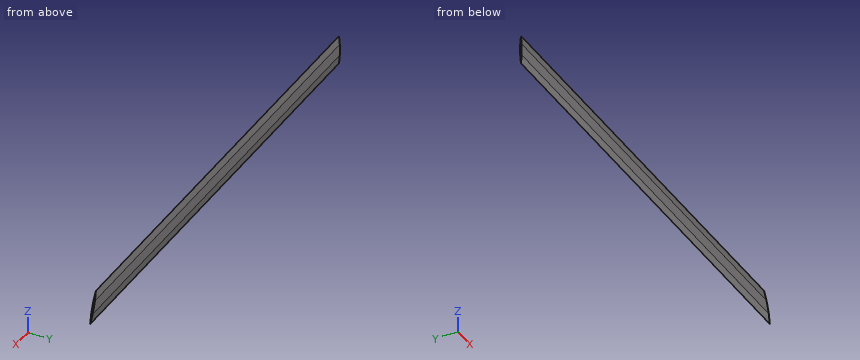
```python
from build123d import *

# Parameters (mm, degrees)
BOSS_EXTRUDE1_DEPTH = 1
CHAMFER1_SIZE       = 0.5
CHAMFER1_SIZE_2     = 6
CHAMFER2_SIZE       = 6
CHAMFER2_SIZE_2     = 0.5


with BuildPart() as part:
    # Sketch1 → Boss-Extrude1 (new body)
    with BuildSketch(Plane(origin=(0, 0, 0), x_dir=(1, 0, 0), z_dir=(0, 1, 0))):
        Polygon((0, -20), (0, 0), (320, 0), (312.720595315, -20), align=None)
    extrude(amount=BOSS_EXTRUDE1_DEPTH)

    # Chamfer1
    # the kernel refuses this chamfer: 6, 0.5 mm, written as the material it takes off along each edge
    with BuildSketch(Plane(origin=(-15.598007041, 0, 0), x_dir=(0, 0.908488621033374, -0.4179095900465534), z_dir=(1, 0, 0))) as chamfer1_piece_1:
        Polygon((CHAMFER1_SIZE * 0.908488621033, CHAMFER1_SIZE * 0.417909590047), (-CHAMFER1_SIZE_2 * 0.417909590047, CHAMFER1_SIZE_2 * 0.908488621033), (0, 0), align=None)
    extrude(amount=351.196014082, mode=Mode.SUBTRACT)
    with BuildSketch(Plane(origin=(-15.598007041, 1, 0), x_dir=(0, -0.908488621033374, -0.4179095900465534), z_dir=(1, 0, 0))) as chamfer1_piece_2:
        Polygon((CHAMFER1_SIZE * 0.908488621033, -CHAMFER1_SIZE * 0.417909590047), (-CHAMFER1_SIZE_2 * 0.417909590047, -CHAMFER1_SIZE_2 * 0.908488621033), (0, 0), align=None)
    extrude(amount=351.196014082, mode=Mode.SUBTRACT)

    # Chamfer2
    # the kernel refuses this chamfer: 6, 0.5 mm, written as the material it takes off along each edge
    with BuildSketch(Plane(origin=(328.318602356, 0, 20), x_dir=(0, -0.0031944650224573633, -0.9999948976835933), z_dir=(-1, 0, 0))) as chamfer2_piece_1:
        Polygon((CHAMFER2_SIZE * 0.999994897684, -CHAMFER2_SIZE * 0.00319446502246), (-CHAMFER2_SIZE_2 * 0.00319446502246, -CHAMFER2_SIZE_2 * 0.999994897684), (0, 0), align=None)
    extrude(amount=343.916609397, mode=Mode.SUBTRACT)
    with BuildSketch(Plane(origin=(328.318602356, 1, 20), x_dir=(0, 0.0031944650224573715, -0.9999948976835933), z_dir=(-1, 0, 0))) as chamfer2_piece_2:
        Polygon((CHAMFER2_SIZE * 0.999994897684, CHAMFER2_SIZE * 0.00319446502246), (-CHAMFER2_SIZE_2 * 0.00319446502246, CHAMFER2_SIZE_2 * 0.999994897684), (0, 0), align=None)
    extrude(amount=343.916609397, mode=Mode.SUBTRACT)


solid = part.part
```
Geometry check sheet. Reference: the model listing, model coordinates, mm. Give positions to 0.01 mm unless a question says otherwise; leave off trailing zeros. Write each loop counter-clockwise with the first axis right and the second up, starting at its lowest first coordinate (ties: lowest second). Pieces come first, ordered by that corner, then holes.
1) Section check A-A, the plane x = 263. Record the boundary of the cut face in (y, z), and give its area (3 significant figures).
2) Material ranges on L1, parallel to Y at x = 22, z = 5.5; L2, parallel to Y at x = 240, z = 16; L3, parallel to X at y = 0.5, z = 16.5, recorded low to high.
3) Section check B-B, the plane y = 0.3. Record the boundary of the cut face in (x, z), and give its area (3 significant figures).
Computed:
1. outline: (0, 6) - (0.5, 0) - (1, 6) - (1, 14) - (0.5, 20) - (0, 14) - close
1. area: 14.0 mm2
2. L1: y = 0.04 to 0.96
2. L2: y = 0.17 to 0.83
2. L3: x = 0 to 313.99
3. outline: (0, 2.4) - (319.13, 2.4) - (313.59, 17.6) - (0, 17.6) - close
3. area: 4,810 mm2
